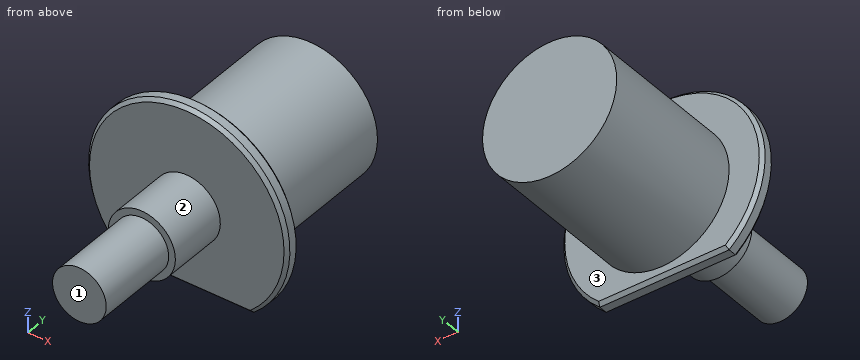
from build123d import *

# Parameters (mm, degrees)
F2_W     = 60
F2_H     = 10
F3_DEPTH = 92.501
F4_SIZE  = 1


with BuildPart() as f1:
    # F0 (on Right) → F1 (revolve)
    with BuildSketch(Plane.YZ):
        Polygon((92.5, 0), (0, 0), (0, -8), (25, -8), (25, -10), (43, -10), (43, -30), (47.5, -30), (47.5, -20), (92.5, -20), align=None)
    revolve(axis=Axis((0, 37.79896, 0), (0, 1, 0)))

    # F2 (on Front) → F3 (cut, through all)
    with BuildSketch(Plane.XZ):
        with Locations((0, -28)):
            Rectangle(F2_W, F2_H)
    extrude(amount=-F3_DEPTH, mode=Mode.SUBTRACT)

    # F4
    f4_edges = [f1.edges().sort_by_distance(p)[0] for p in [
        (0, 47.5, 30),
        (0, 47.5, -23),
        (0, 43, 30),
        (0, 43, -23),
    ]]
    chamfer(f4_edges, length=F4_SIZE)


solid = f1.part
Model file for the job. Use its own axes, mm. Face numbers are marked on the shaded views. A direction names the side the tool comes from. Coordinates: 2 decimals unless noted, no trailing zeros. Loops run counter-clockwise (first coordinate to the right, second up) from the corner with the lowest first, then second, coordinate; pieces in that order, holes last. Notation, with made-up numbers: (10.5, 67.25) -> (23.5, 67.25) arc R24 ccw to (23.5, 102.25) -> close; hole circle Ø6 at (28, -36). An arc over 180 degrees is marked (long way). Use one line per item in the form item = value. Start each with the question number.
(1) Tool access for the marked faces 1, 2 and 3: list every direction of +Z, -Z, +X, -X, +Y, -Y with a clear straight run to the whole face (end or side of a thin tool).
(2) Probe probe 1 along Y at (x, z) = (-17.5, 6); probe 2 along Y at (x, z) = (-7.5, 25); probe 3 along Z at (x, y) = (0, 8). List the from-to ranges inside material, lowest first. Write a range as from..to.
(3) Cut at B-B on y = 72. Give the cut face in (x, z), and give its area (3 significant figures).
(4) Cut at A-A on x = 0. Give the cut face in (y, z), and give its area (3 significant figures).
(5) Flat gauge pins, fed straight in: pin 1 (1 mm diameter, centred on y = 59, z = 19, fed in from +X); pin 2 (10 mm diameter, centred on x = 16.5, z = -2, fed in from -Y); pin 3 (2 mm diameter, centred on x = -21, y = 43, fed in from -Z). Where does each tip first touch, or does it go through?
(6) Cut at C-C on y = 36. Give the cut face in (x, z).
Values:
q1.face_1 = +Z, -Z, +X, -X, -Y
q1.face_2 = -Y
q1.face_3 = +Y
q2.probe_1 = 43..92.5
q2.probe_2 = 43..47.5
q2.probe_3 = -8..8
q3.outline = circle Ø40 at (0, 0)
q3.area = 1,260 mm2
q4.outline = (0, -8) -> (25, -8) -> (25, -10) -> (43, -10) -> (43, -22) -> (44, -23) -> (46.5, -23) -> (47.5, -22) -> (47.5, -20) -> (92.5, -20) -> (92.5, 20) -> (47.5, 20) -> (47.5, 29) -> (46.5, 30) -> (44, 30) -> (43, 29) -> (43, 10) -> (25, 10) -> (25, 8) -> (0, 8) -> close
q4.area = 2,800 mm2
q5.pin_1 = 7.6
q5.pin_2 = 43
q5.pin_3 = -21.72
q6.outline = circle Ø20 at (0, 0)
